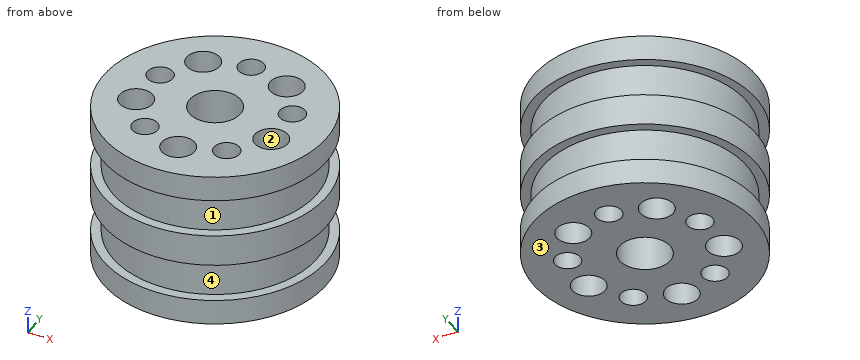
```python
from build123d import *

# Parameters (mm, degrees)
F0_R     = 17.495
F0_R_2   = 15.95
F0_R_3   = 2
F0_R_4   = 2.6
F0_R_5   = 4
F1_DEPTH = 12.5
F3_START = -4
F2_R     = 17.495
F2_R_2   = 16
F3_DEPTH = 6
F5_START = -4
F4_R     = 17.495
F4_R_2   = 16
F5_DEPTH = 6


with BuildPart() as f1:
    # F0 (on Top) → F1 (new body, symmetric)
    with BuildSketch(Plane.XY):
        Circle(F0_R)
        Circle(F0_R_2, mode=Mode.SUBTRACT)
        Circle(F0_R_2)
        with Locations((-6.4656377752, -8.8991869381)):
            Circle(F0_R_3, mode=Mode.SUBTRACT)
        with Locations((-10.6898752432, -3.4733510168)):
            Circle(F0_R_4, mode=Mode.SUBTRACT)
        with Locations((0, -11.24)):
            Circle(F0_R_4, mode=Mode.SUBTRACT)
        with Locations((6.4656377752, -8.8991869381)):
            Circle(F0_R_3, mode=Mode.SUBTRACT)
        with Locations((10.6898752432, -3.4733510168)):
            Circle(F0_R_4, mode=Mode.SUBTRACT)
        with Locations((-10.4616216792, 3.3991869381)):
            Circle(F0_R_3, mode=Mode.SUBTRACT)
        with Locations((-6.6067062358, 9.0933510168)):
            Circle(F0_R_4, mode=Mode.SUBTRACT)
        Circle(F0_R_5, mode=Mode.SUBTRACT)
        with Locations((10.4616216792, 3.3991869381)):
            Circle(F0_R_3, mode=Mode.SUBTRACT)
        with Locations((0, 11)):
            Circle(F0_R_3, mode=Mode.SUBTRACT)
        with Locations((6.6067062358, 9.0933510168)):
            Circle(F0_R_4, mode=Mode.SUBTRACT)
    extrude(amount=F1_DEPTH, both=True)

    # F2 (on face) → F3 (cut)
    with BuildSketch(Plane.XY.offset(12.5).offset(F3_START)):
        Circle(F2_R)
        Circle(F2_R_2, mode=Mode.SUBTRACT)
    extrude(amount=-F3_DEPTH, mode=Mode.SUBTRACT)

    # F4 (on face) → F5 (cut)
    with BuildSketch(Plane(origin=(0, 0, -12.5), x_dir=(1, 0, 0), z_dir=(0, 0, -1)).offset(F5_START)):
        Circle(F4_R)
        Circle(F4_R_2, mode=Mode.SUBTRACT)
    extrude(amount=-F5_DEPTH, mode=Mode.SUBTRACT)


solid = f1.part
```
Model file for the job. Use its own axes, mm. Face numbers are marked on the shaded views. Round coordinates to 2 decimals unless told otherwise and drop trailing zeros. Write each loop counter-clockwise with the first axis right and the second up, starting at its lowest first coordinate (ties: lowest second). Pieces come first, ordered by that corner, then holes. Notation, with made-up numbers: (54.5, 45.5) - (78.5, 45.5) arc R26 cw to (78.5, 69.5) - close; hole circle Ø6 at (13, -37.75). An arc over 180 degrees is marked (long way). Use CSV: the item, a comma, the result in double quotes. Start each with the question number.
Item 1: Band-saw the part on B-B (y = 0). Write the cut outline in (x, z) (3 decimals), and give its area (3 significant figures).
Item 2: Pin check, flat tips, straight feed: P1, Ø12, axis at y = -0.5, z = -8.5, coming from the +X side (3 decimals); P2, Ø3, axis at x = 7.5, z = -5, coming from the -Y side; P3, Ø4, axis at x = -12, z = 3, coming from the -Y side; P4, Ø2, axis at y = -13.5, z = -4, coming from the +X side. Stop position of each tip, or through.
Item 3: Two-plate mould, pull along Z, no slides. Class the marked faces 1, 2, 3 and 4: released by +Z, released by -Z, zero draft, split by the parting line, or undercut.
Item 4: Band-saw the part on A-A (x = 0). State how many separate pieces and enclosed holes the cut face has, and give its area (3 significant figures).
Item 5: Drill centre lines: L1, parallel to Y at x = 0, z = -10.5 (3 decimals); L2, parallel to Y at x = 0, z = 2.75; L3, parallel to X at y = 7, z = 3. Where is each one in solid material? Low to high. Write a range as [from, to].
Checked values:
1,outline,"(-17.495, -12.5) - (-4, -12.5) - (-4, 12.5) - (-17.495, 12.5) - (-17.495, 8.5) - (-16, 8.5) - (-16, 2.5) - (-17.495, 2.5) - (-17.495, -2.5) - (-16, -2.5) - (-16, -8.5) - (-17.495, -8.5) - close; (4, -12.5) - (17.495, -12.5) - (17.495, -8.5) - (16, -8.5) - (16, -2.5) - (17.495, -2.5) - (17.495, 2.5) - (16, 2.5) - (16, 8.5) - (17.495, 8.5) - (17.495, 12.5) - (4, 12.5) - close"
1,area,"639 mm²"
2,P1,"stops at x = 17.495"
2,P2,"stops at y = -14.83"
2,P3,"stops at y = -14.31"
2,P4,"stops at x = 9.99"
3,face 1,"undercut"
3,face 2,"zero draft"
3,face 3,"released by -Z"
3,face 4,"undercut"
4,separate pieces,"4"
4,enclosed holes,"0"
4,area,"409 mm²"
5,L1,"y = [-17.495, -13.84], [-8.64, -4], [4, 9], [13, 17.495]"
5,L2,"y = [-16, -13.84], [-8.64, -4], [4, 9], [13, 16]"
5,L3,"x = [-14.39, -8.15], [-5.06, 5.06], [8.15, 14.39]"
